Check sheet for the modelled part. Datum: model origin and axes. Units: mm. Round coordinates to 2 decimals unless told otherwise and drop trailing zeros. Order: outer loops, then holes, each group sorted by start corner. A loop starts at its lowest first (then second) coordinate and runs counter-clockwise, first axis right, second up. Notation, with made-up numbers: (36.25, -35.75) -> (73.25, -35.75) arc R19 ccw to (73.25, 1.25) -> close; hole circle Ø1 at (-21, -25). An arc over 180 degrees is marked (long way). Use CSV: the item, a comma, the result in double quotes.
```python
from build123d import *

# Parameters (mm, degrees)
SKETCH1_W           = 100
SKETCH1_H           = 100
BOSS_EXTRUDE1_DEPTH = 10
CUT_EXTRUDE1_REACH  = 73.414
SKETCH2_R           = 2.5
SKETCH3_R           = 2.5
CUT_EXTRUDE2_DEPTH  = 20
FILLET2_R           = 25
FILLET3_R           = 25


with BuildPart() as part:
    # Sketch1 → Boss-Extrude1 (new body)
    with BuildSketch(Plane.XY):
        Rectangle(SKETCH1_W, SKETCH1_H)
    extrude(amount=BOSS_EXTRUDE1_DEPTH)

    # Sketch2 → Cut-Extrude1 (cut, up to next)
    with BuildSketch(Plane(origin=(0, 0, 0), x_dir=(-1, 0, 0), z_dir=(0, 0, -1)), mode=Mode.PRIVATE) as cut_extrude1_sk1:
        with Locations((0, -5)):
            Circle(SKETCH2_R)
    cut_extrude1_tool1 = extrude(cut_extrude1_sk1.sketch, amount=-CUT_EXTRUDE1_REACH, mode=Mode.PRIVATE) & part.part
    # Sketch2 → Cut-Extrude1 (cut, up to next)
    with BuildSketch(Plane(origin=(0, 0, 0), x_dir=(-1, 0, 0), z_dir=(0, 0, -1)), mode=Mode.PRIVATE) as cut_extrude1_sk2:
        with BuildLine():
            ThreePointArc((37.5, 0), (0, 37.5), (-37.5, 0))
            ThreePointArc((-37.5, 0), (-35, -2.5), (-32.5, 0))
            ThreePointArc((-32.5, 0), (0, 32.5), (32.5, 0))
            ThreePointArc((32.5, 0), (35, -2.5), (37.5, 0))
        make_face()
    cut_extrude1_tool2 = extrude(cut_extrude1_sk2.sketch, amount=-CUT_EXTRUDE1_REACH, mode=Mode.PRIVATE) & part.part
    add(cut_extrude1_tool1.solids().sort_by_distance((0, -5, 0))[0], mode=Mode.SUBTRACT)
    add(cut_extrude1_tool2.solids().sort_by_distance((0, 33.35, 0))[0], mode=Mode.SUBTRACT)

    # Sketch3 → Cut-Extrude2 (cut)
    with BuildSketch(Plane.XZ.offset(50)):
        with Locations((-35, 5)):
            Circle(SKETCH3_R)
        with Locations((0, 5)):
            Circle(SKETCH3_R)
        with Locations((35, 5)):
            Circle(SKETCH3_R)
    extrude(amount=-CUT_EXTRUDE2_DEPTH, mode=Mode.SUBTRACT)

    # Fillet2
    fillet2_edges = [part.edges().sort_by_distance(p)[0] for p in [
        (-50, 50, 5),
    ]]
    fillet(fillet2_edges, radius=FILLET2_R)

    # Fillet3
    fillet3_edges = [part.edges().sort_by_distance(p)[0] for p in [
        (50, 50, 5),
    ]]
    fillet(fillet3_edges, radius=FILLET3_R)


solid = part.part
```
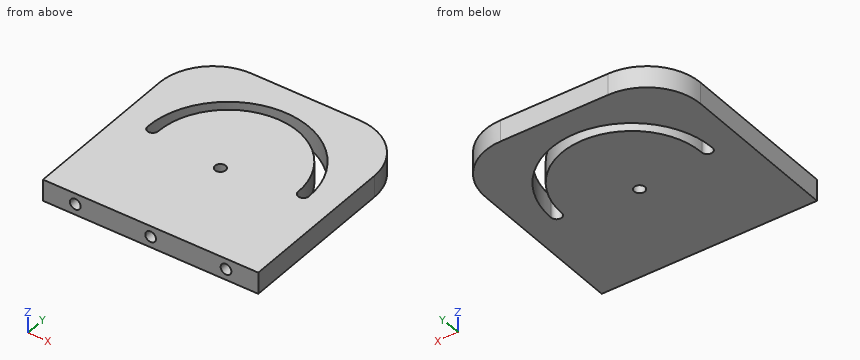
Q1. Go/stop test with flat-tipped pins: pin 1 (2.5 mm diameter, centred on x = -35, z = 6, fed in from -Y); pin 2 (6 mm diameter, centred on x = 35, z = 5, fed in from +Y); pin 3 (1 mm diameter, centred on y = 31.5, z = 4.5, fed in from -X). Record where each tip stops, or that it passes through.
Result sheet:
pin 1,"stops at y = -30"
pin 2,"stops at y = 49"
pin 3,"stops at x = -49.27"
Q2. Sectioned sample at A-A, the plane y = -5. Enter the section's corners in (x, z), then the cut area to 3 significant figures.
Result sheet:
outline,"(-50, 0) -> (-2.5, 0) -> (-2.5, 10) -> (-50, 10) -> close; (2.5, 0) -> (50, 0) -> (50, 10) -> (2.5, 10) -> close"
area,"950 mm^2"
Q3. Scan lines: L1, parallel to Y at x = 0, z = 3; L2, parallel to X at y = 18.5, z = 3.5; L3, parallel to X at y = 9.5, z = 2. Record each from-to range of solid material in increasing order.
Result sheet:
L1,"y = -30 to -7.5, -2.5 to 32.5, 37.5 to 50"
L2,"x = -50 to -32.62, -26.72 to 26.72, 32.62 to 50"
L3,"x = -50 to -36.28, -31.08 to 31.08, 36.28 to 50"
Q4. Sectioned sample at C-C, the plane z = 8.75. Enter the section's corners in (x, y), then the cut area to 3 significant figures.
Result sheet:
outline,"(-50, -50) -> (50, -50) -> (50, 25) arc R25 ccw to (25, 50) -> (-25, 50) arc R25 ccw to (-50, 25) -> close; hole (-37.5, 0) arc R2.5 ccw to (-32.5, 0) arc R32.5 cw to (32.5, 0) arc R2.5 ccw to (37.5, 0) arc R37.5 ccw to start; hole circle Ø5 at (0, -5)"
area,"9,140 mm^2"
Q5. Sectioned sample at D-D, the plane y = 21. Enter the section's corners in (x, z).
Result sheet:
outline,"(-50, 0) -> (-31.07, 0) -> (-31.07, 10) -> (-50, 10) -> close; (-24.8, 0) -> (24.8, 0) -> (24.8, 10) -> (-24.8, 10) -> close; (31.07, 0) -> (50, 0) -> (50, 10) -> (31.07, 10) -> close"
Q6. Sectioned sample at B-B, the plane x = 0. Enter the section's corners in (y, z).
Result sheet:
outline,"(-50, 0) -> (-7.5, 0) -> (-7.5, 10) -> (-50, 10) -> (-50, 7.5) -> (-30, 7.5) -> (-30, 2.5) -> (-50, 2.5) -> close; (-2.5, 0) -> (32.5, 0) -> (32.5, 10) -> (-2.5, 10) -> close; (37.5, 0) -> (50, 0) -> (50, 10) -> (37.5, 10) -> close"
